Geometry: final body of the model. Coordinates: model frame, mm. Face numbers are marked on the shaded views. A direction names the side the tool comes from. Coordinates: 2 decimals unless noted, no trailing zeros. Order: outer loops, then holes, each group sorted by start corner. A loop starts at its lowest first (then second) coordinate and runs counter-clockwise, first axis right, second up. Notation, with made-up numbers: (-17.5, 5) - (28.5, 5) arc R15 ccw to (28.5, 25) - close; hole circle Ø11 at (69.25, 72). An arc over 180 degrees is marked (long way). Use a Markdown table: item, result. Add a question column.
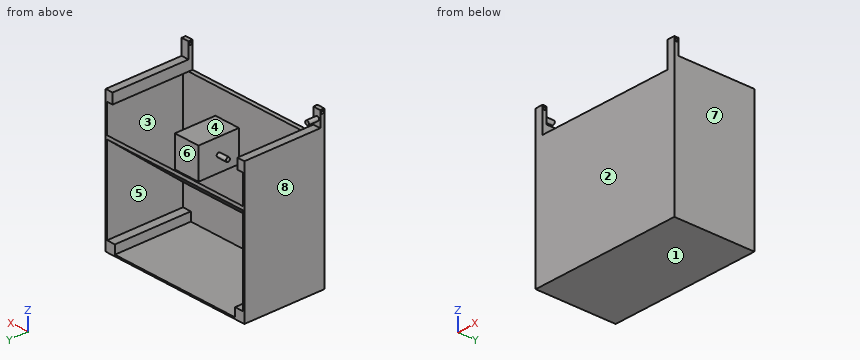
```python
from build123d import *

# Parameters (mm, degrees)
BOSS_EXTRUDE1_DEPTH     = 8
CUT_EXTRUDE1_DEPTH      = 213.282830205
CUT_EXTRUDE1_DEPTH_BACK = 213.282830205
SKETCH2_R               = 2.5
SKETCH3_W               = 20
SKETCH3_H               = 20
SKETCH3_W_2             = 15
BOSS_EXTRUDE2_DEPTH     = 150
BOSS_EXTRUDE3_DEPTH     = 150
SKETCH5_W               = 51
SKETCH5_H               = 60
BOSS_EXTRUDE4_DEPTH     = 80
SKETCH7_R               = 4
BOSS_EXTRUDE5_DEPTH     = 20
BOSS_EXTRUDE6_REACH     = 372.761
SKETCH9_R               = 4
BOSS_EXTRUDE7_DEPTH     = 20


with BuildPart() as part:
    # Sketch1 → Boss-Extrude1 (new body)
    with BuildSketch(Plane(origin=(0, 0, 0), x_dir=(1, 0, 0), z_dir=(0, 1, 0))):
        Polygon((135, -150), (150, -150), (150, 150), (-150, 150), (-150, -150), (-135, -150), (-135, -100), (135, -100), align=None)
    extrude(amount=BOSS_EXTRUDE1_DEPTH)

    # Sketch2 → Cut-Extrude1 (cut, two sides: drawn at the far end of the back side and taken through both)
    with BuildSketch(Plane(origin=(0, 0, 0), x_dir=(0, 0, -1), z_dir=(1, 0, 0)).offset(-CUT_EXTRUDE1_DEPTH_BACK)):
        with Locations((-145.033528283, 4)):
            Circle(SKETCH2_R)
    extrude(amount=CUT_EXTRUDE1_DEPTH + CUT_EXTRUDE1_DEPTH_BACK, mode=Mode.SUBTRACT)

    # Sketch3 → Boss-Extrude2 (add)
    with BuildSketch(Plane(origin=(0, 8, 0), x_dir=(1, 0, 0), z_dir=(0, 1, 0))):
        with Locations((-140, 140)):
            Rectangle(SKETCH3_W, SKETCH3_H)
        with Locations((140, 140)):
            Rectangle(SKETCH3_W, SKETCH3_H)
        with Locations((142.5, -110)):
            Rectangle(SKETCH3_W_2, SKETCH3_H)
        with Locations((-142.5, -110)):
            Rectangle(SKETCH3_W_2, SKETCH3_H)
    extrude(amount=BOSS_EXTRUDE2_DEPTH)

    # Sketch4 → Boss-Extrude3 (add)
    with BuildSketch(Plane(origin=(0, 8, 0), x_dir=(1, 0, 0), z_dir=(0, 1, 0))):
        Polygon((-147, 147), (-147, -117), (-150, -120), (-150, 150), (150, 150), (150, -120), (147, -117), (147, 147), align=None)
    extrude(amount=BOSS_EXTRUDE3_DEPTH)

    # Sketch5 → Boss-Extrude4 (add)
    with BuildSketch(Plane(origin=(0, 8, 0), x_dir=(1, 0, 0), z_dir=(0, 1, 0))):
        with Locations((51.38892732, -20)):
            Rectangle(SKETCH5_W, SKETCH5_H)
    extrude(amount=BOSS_EXTRUDE4_DEPTH)

    # Sketch7 → Boss-Extrude5 (add)
    with BuildSketch(Plane.ZY.offset(-25.88892732)):
        with Locations(Location((20.016570429, 48, 0), (0, 0, 180))):
            Circle(SKETCH7_R)
    extrude(amount=BOSS_EXTRUDE5_DEPTH)

    # Sketch8 → Boss-Extrude6 (add, up to next)
    with BuildSketch(Plane.ZY.offset(150), mode=Mode.PRIVATE) as boss_extrude6_sk1:
        Polygon((37.367547096, 158), (-94.778166859, 0), (-87.891172035, 0), (44.254541919, 158), align=None)
    boss_extrude6_tool1 = extrude(boss_extrude6_sk1.sketch, amount=-BOSS_EXTRUDE6_REACH, mode=Mode.PRIVATE) - part.part
    add(boss_extrude6_tool1.solids().sort_by_distance((-150, 79, -25.261812))[0])

    # Sketch9 → Boss-Extrude7 (add)
    with BuildSketch(Plane(origin=(0, 8, 0), x_dir=(1, 0, 0), z_dir=(0, 1, 0))):
        with Locations(Location((-143.273126196, -133.426649838, 0), (0, 0, 270))):
            Circle(SKETCH9_R)
    extrude(amount=BOSS_EXTRUDE7_DEPTH)


solid = part.part
```
1) Pin query (flat end, axial travel): pin 1 (10 mm diameter, centred on x = -63.5, z = -40.5, fed in from +Y); pin 2 (1 mm diameter, centred on x = 78.5, z = 66.5, fed in from +Y); pin 3 (1 mm diameter, centred on x = 45, z = -83, fed in from -Y); pin 4 (4 mm diameter, centred on x = -142, z = 134, fed in from +Y). Return the tip coordinate at first contact, or that it passes through.
2) Section B-B (y = 39). Return loops of the section in (x, z).
3) Ray query, line 1 along X through (y, z) = (31, 33); line 2 along X through (y, z) = (117, 13.5); line 3 along Z through (x, y) = (140.25, 4). Return the intervals inside material, ascending.
4) Section D-D (z = -47.5). Return loops of the section in (x, y).
5) Section C-C (x = -116.5). Return loops of the section in (y, z), then the cut area to 3 significant figures.
6) Draft query along Y for the marked faces 1, 2 and 3. Return one class per face: pulls with the +Y half, pulls with the -Y half, needs draft (parallel to the pull), parting line crosses it, or undercut.
7) Section A-A (z = 113). Return loops of the section in (x, y).
8) Set-up query: the marked faces 4, 5, 6, 7 and 8. Return all of +Z, -Z, +X, -X, +Y, -Y with unobstructed straight access to the full face (end or side cutting, diameter ignored); none if empty.
Values follow:
| question | item | result |
|---|---|---|
| 1 | pin 1 | stops at y = 70.88 |
| 1 | pin 2 | stops at y = 8 |
| 1 | pin 3 | stops at y = 0 |
| 1 | pin 4 | stops at y = 28 |
| 2 | outline | (-150, -150) - (150, -150) - (150, 120) - (135, 120) - (135, 100) - (147, 100) - (147, -55.27) - (-147, -55.27) - (-147, 100) - (-135, 100) - (-135, 120) - (-150, 120) - close; (25.89, -10) - (76.89, -10) - (76.89, 50) - (25.89, 50) - close; hole (-147, -130) - (-130, -130) - (-130, -147) - (130, -147) - (130, -130) - (147, -130) - (147, -62.16) - (-147, -62.16) - close |
| 3 | line 1 | x = -150 to -147, 25.89 to 76.89, 147 to 150 |
| 3 | line 2 | x = -150 to -147, 147 to 150 |
| 3 | line 3 | z = -150 to 142.53, 147.53 to 150 |
| 4 | outline | (-150, 0) - (150, 0) - (150, 158) - (147, 158) - (147, 56.53) - (-147, 56.53) - (-147, 158) - (-150, 158) - close; hole (-147, 8) - (147, 8) - (147, 48.29) - (-147, 48.29) - close |
| 5 | outline | (0, -150) - (158, -150) - (158, -147) - (8, -147) - (8, -88.09) - (158, 37.37) - (158, 44.25) - (8, -81.2) - (8, 100) - (0, 100) - close |
| 5 | area | 3,480 mm² |
| 6 | face 1 | needs draft |
| 6 | face 2 | pulls with the -Y half |
| 6 | face 3 | undercut |
| 7 | outline | (-150, 0) - (-135, 0) - (-135, 158) - (-150, 158) - close; (135, 0) - (150, 0) - (150, 158) - (135, 158) - close |
| 8 | face 4 | +Z, +Y |
| 8 | face 5 | +Y |
| 8 | face 6 | +Z |
| 8 | face 7 | +Z, -Z, +X, +Y, -Y |
| 8 | face 8 | +Z, -Z, -X, +Y, -Y |
